Geometry check sheet. Reference: the model listing, model coordinates, mm. Coordinates: 2 decimals unless noted, no trailing zeros. Write each loop counter-clockwise with the first axis right and the second up, starting at its lowest first coordinate (ties: lowest second). Pieces come first, ordered by that corner, then holes. Notation, with made-up numbers: (29.5, 25.25) -> (53.5, 25.25) arc R13 cw to (53.5, 34.25) -> close; hole circle Ø9 at (-6, 43.25). An arc over 180 degrees is marked (long way). Answer in a Markdown table with one row per item. Add a question column.
1. Cross-section at C-C on x = 12. Record the cut outline in (y, z).
2. Cross-section at D-D on y = -109. Record the cut outline in (x, z), and give its area (3 significant figures).
3. Cross-section at A-A on x = -5. Record the cut outline in (y, z), and give its area (3 significant figures).
4. Cross-section at B-B on y = -90.5. Record the cut outline in (x, z).
5. Scan lines: L1, parallel to X at y = -113.5, z = 0.05; L2, parallel to X at y = -120, z = 0.05; L3, parallel to Y at x = 21.5, z = 0.05. Record each from-to range of solid material in increasing order. Write a range as from..to.
```python
from build123d import *
from OCP.BRepFilletAPI import BRepFilletAPI_MakeChamfer

# Parameters (mm, degrees)
SKETCH2_R           = 1.5875
BOSS_EXTRUDE1_DEPTH = 0.118
SKETCH3_R           = 2
CUT_EXTRUDE1_DEPTH  = 267.27056526
CHAMFER1_SIZE       = 20
CHAMFER1_SIZE2      = 24.415491775
SKETCH4_W           = 440.908945527
SKETCH4_H           = 173.352966469
CUT_EXTRUDE4_DEPTH  = 251.000027848
SKETCH5_W           = 18
SKETCH5_H           = 18
SKETCH5_R           = 2
BOSS_EXTRUDE2_DEPTH = 0.118
FILLET1_R           = 0.25


with BuildPart() as part:
    # Sketch2 → Boss-Extrude1 (new body)
    with BuildSketch(Plane.XY):
        with BuildLine():
            Line((99.563224144, -21.926473835), (48.69, -83.15))
            ThreePointArc((48.69, -83.15), (13.462751156, -108.648946204), (0, -150))
            ThreePointArc((0, -150), (-13.462751156, -108.648946204), (-48.69, -83.15))
            Line((-48.69, -83.15), (-99.563224144, -21.926473835))
            Line((-99.563224144, -21.926473835), (-140, -21.926473835))
            ThreePointArc((-140, -21.926473835), (-145.965681261, -3.736597624), (-158.952536164, 10.327631798))
            Line((-158.952536164, 10.327631798), (-220, 53.073526165))
            Line((-220, 53.073526165), (-67, 53.073526165))
            ThreePointArc((-67, 53.073526165), (-51.137889855, 23.094319589), (-17.95554779, 16.073526165))
            Line((-17.95554779, 16.073526165), (-15.117733438, 43.073526165))
            Line((-15.117733438, 43.073526165), (-12, 30.568980335))
            ThreePointArc((-12, 30.568980335), (0, 33.073526165), (12, 30.568980335))
            Line((12, 30.568980335), (15.117733438, 43.073526165))
            Line((15.117733438, 43.073526165), (17.95554779, 16.073526165))
            ThreePointArc((17.95554779, 16.073526165), (51.137889855, 23.094319589), (67, 53.073526165))
            Line((67, 53.073526165), (220, 53.073526165))
            Line((220, 53.073526165), (158.952536164, 10.327631798))
            ThreePointArc((158.952536164, 10.327631798), (145.965681261, -3.736597624), (140, -21.926473835))
            Line((140, -21.926473835), (99.563224144, -21.926473835))
        make_face()
        with Locations((46.19, 13)):
            Circle(SKETCH2_R, mode=Mode.SUBTRACT)
        with Locations((-46.19, 13)):
            Circle(SKETCH2_R, mode=Mode.SUBTRACT)
        with Locations((46.19, -80.65)):
            Circle(SKETCH2_R, mode=Mode.SUBTRACT)
        with Locations((-46.19, -80.65)):
            Circle(SKETCH2_R, mode=Mode.SUBTRACT)
    extrude(amount=BOSS_EXTRUDE1_DEPTH)

    # Sketch3 → Cut-Extrude1 (cut, through all)
    with BuildSketch(Plane(origin=(0, 0, 0), x_dir=(-1, 0, 0), z_dir=(0, 0, -1))):
        with Locations((165, 49.573526165)):
            Circle(SKETCH3_R)
        with Locations((165, 19.573526165)):
            Circle(SKETCH3_R)
        with Locations((150, 34.573526165)):
            Circle(SKETCH3_R)
    cut_extrude1 = extrude(amount=-CUT_EXTRUDE1_DEPTH, mode=Mode.SUBTRACT)

    # Mirror2: Cut-Extrude1 across plane
    add(cut_extrude1.mirror(Plane(origin=(0, 0, 0), x_dir=(0, 0, 1), z_dir=(1, 0, 0))), mode=Mode.SUBTRACT)

    # Chamfer1: one chamfer whose edges measure the first distance from different faces: ONE call of the kernel's chamfer builder (chamfer() names one face for all edges)
    chamfer1_edges_1 = [part.edges().sort_by_distance(p)[0] for p in [
        (220, 53.073526165, 0.059),
    ]]
    chamfer1_side_1 = [part.faces().sort_by_distance(p)[0] for p in [
        (143.5, 53.073526165, 0.059),
    ]]
    chamfer1_edges_2 = [part.edges().sort_by_distance(p)[0] for p in [
        (-220, 53.073526165, 0.059),
    ]]
    chamfer1_side_2 = [part.faces().sort_by_distance(p)[0] for p in [
        (-143.5, 53.073526165, 0.059),
    ]]
    chamfer1 = BRepFilletAPI_MakeChamfer(part.part.solid().wrapped)
    for e in chamfer1_edges_1:
        chamfer1.Add(CHAMFER1_SIZE, CHAMFER1_SIZE2, e.wrapped, chamfer1_side_1[0].wrapped)  # the first distance lies on this face
    for e in chamfer1_edges_2:
        chamfer1.Add(CHAMFER1_SIZE, CHAMFER1_SIZE2, e.wrapped, chamfer1_side_2[0].wrapped)  # the first distance lies on this face
    add(Compound.cast(chamfer1.Shape()), mode=Mode.REPLACE)

    # Sketch4 → Cut-Extrude4 (cut, through all)
    with BuildSketch(Plane(origin=(0, 0, 0), x_dir=(-1, 0, 0), z_dir=(0, 0, -1))):
        with Locations((-5.514300507, -5.754470648)):
            Rectangle(SKETCH4_W, SKETCH4_H)
    extrude(amount=-CUT_EXTRUDE4_DEPTH, mode=Mode.SUBTRACT)

    # Sketch5 → Boss-Extrude2 (add)
    with BuildSketch(Plane(origin=(0, 0, 0), x_dir=(-1, 0, 0), z_dir=(0, 0, -1))):
        with Locations((0, -83.430953883)):
            Rectangle(SKETCH5_W, SKETCH5_H)
        with Locations((-5, -89.430953883)):
            Circle(SKETCH5_R, mode=Mode.SUBTRACT)
        with Locations((5, -89.430953883)):
            Circle(SKETCH5_R, mode=Mode.SUBTRACT)
        with Locations((-5, -83.430953883)):
            Circle(SKETCH5_R, mode=Mode.SUBTRACT)
        with Locations((5, -83.430953883)):
            Circle(SKETCH5_R, mode=Mode.SUBTRACT)
        with Locations((-5, -77.430953883)):
            Circle(SKETCH5_R, mode=Mode.SUBTRACT)
        with Locations((5, -77.430953883)):
            Circle(SKETCH5_R, mode=Mode.SUBTRACT)
    extrude(amount=-BOSS_EXTRUDE2_DEPTH)

    # Fillet1
    fillet1_edges = [part.edges().sort_by_distance(p)[0] for p in [
        (0, -150, 0.059),
    ]]
    fillet(fillet1_edges, radius=FILLET1_R)


solid = part.part
```
Results found:
| question | item | result |
|---|---|---|
| 1 | outline | (-110.74, 0) -> (-92.43, 0) -> (-92.43, 0.12) -> (-110.74, 0.12) -> close |
| 2 | outline | (-13.21, 0) -> (13.21, 0) -> (13.21, 0.12) -> (-13.21, 0.12) -> close |
| 2 | area | 3.12 mm^2 |
| 3 | outline | (-123.97, 0) -> (-91.43, 0) -> (-91.43, 0.12) -> (-123.97, 0.12) -> close; (-87.43, 0) -> (-85.43, 0) -> (-85.43, 0.12) -> (-87.43, 0.12) -> close; (-81.43, 0) -> (-79.43, 0) -> (-79.43, 0.12) -> (-81.43, 0.12) -> close; (-75.43, 0) -> (-74.43, 0) -> (-74.43, 0.12) -> (-75.43, 0.12) -> close |
| 3 | area | 4.43 mm^2 |
| 4 | outline | (-9, 0) -> (-6.69, 0) -> (-6.69, 0.12) -> (-9, 0.12) -> close; (-3.31, 0) -> (3.31, 0) -> (3.31, 0.12) -> (-3.31, 0.12) -> close; (6.69, 0) -> (9, 0) -> (9, 0.12) -> (6.69, 0.12) -> close |
| 5 | L1 | x = -10.23..10.23 |
| 5 | L2 | x = -6.73..6.73 |
| 5 | L3 | y = -99.42..-92.43 |
